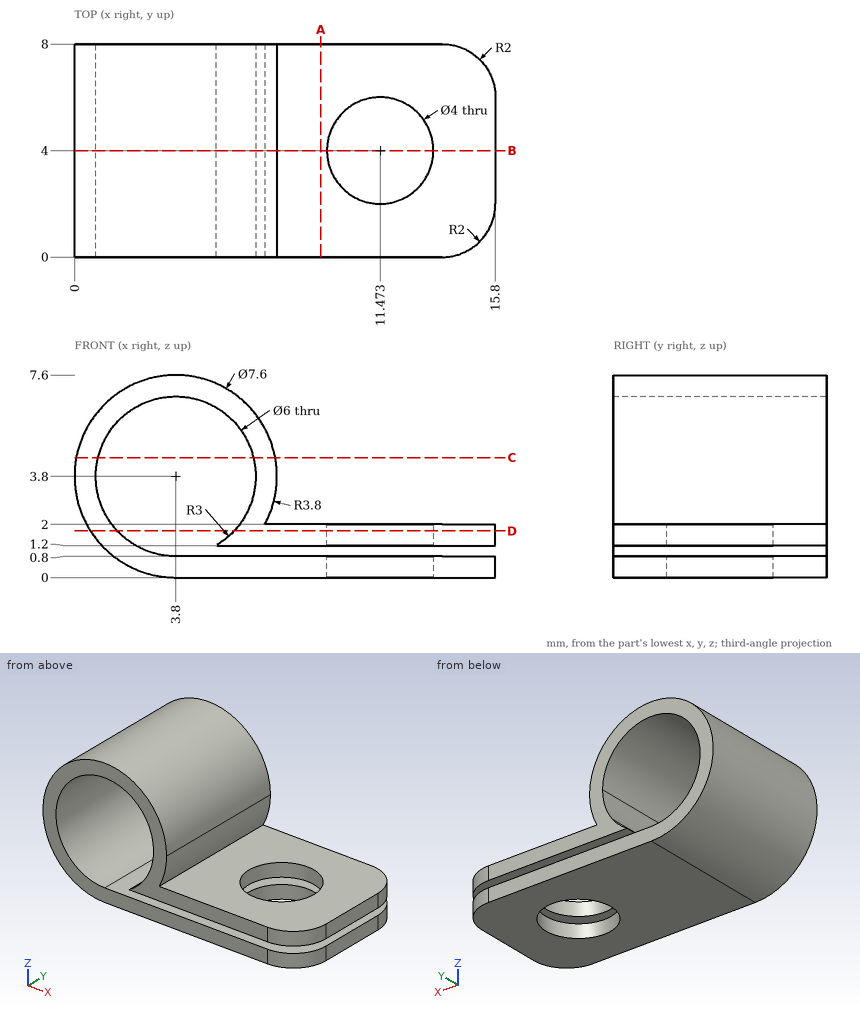
Source: three-view drawing plus pictorial views. Frame: mm from the lowest corner of the part. Give positions to 0.01 mm unless a question says otherwise; leave off trailing zeros. Order: outer loops, then holes, each group sorted by start corner. A loop starts at its lowest first (then second) coordinate and runs counter-clockwise, first axis right, second up. Notation, with made-up numbers: M -17,-26.5 L -12,-26.5 A23 cw -12,-4.5 Z; hole C 7.5,-7.75 d10. An arc over 180 degrees is marked long. Return JSON: item names as keys, results as strings.
Item 1: Cut plane D-D (z = 1.75). Return loops of the section in (x, y).
Solutions:
{"outline": "M 0.6,0 L 1.61,0 L 1.61,8 L 0.6,8 Z; M 5.99,0 L 13.8,0 A2 ccw 15.8,2 L 15.8,6 A2 ccw 13.8,8 L 5.99,8 Z; hole C 11.47,4 d4"}
Item 2: Cut plane B-B (y = 4). Return loops of the section in (x, z).
Solutions:
{"outline": "M 3.8,0 L 9.47,0 L 9.47,0.8 L 3.8,0.8 A3 cw long 5.3,1.2 L 9.47,1.2 L 9.47,2 L 7.15,2 A3.8 ccw long Z; M 13.47,0 L 15.8,0 L 15.8,0.8 L 13.47,0.8 Z; M 13.47,1.2 L 15.8,1.2 L 15.8,2 L 13.47,2 Z"}
Item 3: Ray query, probe 1 along Z at (x, y) = (3.8, 3); probe 2 along Z at (x, y) = (13, 7.75). Return the intervals inside material, ascending.
Solutions:
{"probe 1": "0 to 0.8, 6.8 to 7.6", "probe 2": "0 to 0.8, 1.2 to 2"}
Item 4: Cut plane C-C (z = 4.5). Return loops of the section in (x, y) (1 decimal), then the cut area to 3 significant figures.
Solutions:
{"outline": "M 0.1,0 L 0.9,0 L 0.9,8 L 0.1,8 Z; M 6.7,0 L 7.5,0 L 7.5,8 L 6.7,8 Z", "area": "13.1 mm^2"}
Item 5: Cut plane A-A (x = 9.25). Return loops of the section in (y, z), then the cut area to 3 significant figures.
Solutions:
{"outline": "M 0,0 L 8,0 L 8,0.8 L 0,0.8 Z; M 0,1.2 L 8,1.2 L 8,2 L 0,2 Z", "area": "12.8 mm^2"}
